from build123d import *

# Parameters (mm, degrees)
SKETCH1_R           = 1.6
BOSS_EXTRUDE1_DEPTH = 11
CUT_EXTRUDE1_DEPTH  = 6


with BuildPart() as part:
    # Sketch1 → Boss-Extrude1 (new body)
    with BuildSketch(Plane(origin=(0, 0, 0), x_dir=(1, 0, 0), z_dir=(0, 1, 0))):
        with BuildLine():
            Line((-4.5, -3.6), (4.5, -3.6))
            ThreePointArc((4.5, -3.6), (5.560660172, -3.160660172), (6, -2.1))
            Line((6, -2.1), (6, 2.1))
            ThreePointArc((6, 2.1), (5.560660172, 3.160660172), (4.5, 3.6))
            Line((4.5, 3.6), (-4.5, 3.6))
            ThreePointArc((-4.5, 3.6), (-5.560660172, 3.160660172), (-6, 2.1))
            Line((-6, 2.1), (-6, -2.1))
            ThreePointArc((-6, -2.1), (-5.560660172, -3.160660172), (-4.5, -3.6))
        make_face()
        with Locations((3, 0)):
            Circle(SKETCH1_R, mode=Mode.SUBTRACT)
    extrude(amount=-BOSS_EXTRUDE1_DEPTH)

    # Sketch2 → Cut-Extrude1 (cut)
    with BuildSketch(Plane.ZY.offset(6)):
        Polygon((-0.333384704, -11), (1.1, -11), (1.1, 0), (-0.8, 0), (-0.1, -0.45), (-0.1, -0.85), (-0.8, -1.3), (-0.8, -1.65), (-0.8, -1.999993395), (-0.1, -2.449993395), (-0.1, -2.849993395), (-0.8, -3.299993395), (-0.8, -3.64998679), (-0.8, -3.99998679), (-0.1, -4.44998679), (-0.1, -4.84998679), (-0.8, -5.29998679), (-0.8, -5.649980186), (-0.8, -5.999980186), (-0.1, -6.449980186), (-0.1, -6.849980186), (-0.8, -7.299980186), (-0.8, -7.649973581), (-0.8, -7.999973581), (-0.1, -8.449973581), (-0.1, -8.849973581), (-0.8, -9.299973581), (-0.8, -9.649966976), (-0.8, -9.999966976), (-0.1, -10.449966976), (-0.1, -10.849966976), align=None)
    extrude(amount=-CUT_EXTRUDE1_DEPTH, mode=Mode.SUBTRACT)


solid = part.part
Can you work these out from the model? Positions are in its coordinate system, mm. A direction names the side the tool comes from. Coordinates: 2 decimals unless noted, no trailing zeros. Write each loop counter-clockwise with the first axis right and the second up, starting at its lowest first coordinate (ties: lowest second). Pieces come first, ordered by that corner, then holes. Notation, with made-up numbers: (54, 52.5) - (91, 52.5) arc R18 ccw to (91, 81.5) - close; hole circle Ø9 at (15, 52.5). An arc over 180 degrees is marked (long way). Return JSON: item names as keys, results as strings. Group by question number.
Item 1: If we section it at B-B (y = -3.5): Write out the boundary of the cut face in (x, z), then the cut area to 3 significant figures.
Item 2: I'm going to push a flat-ended pin straight in: pin 1 Ø1.9 at (x, z) = (3, 0) entering from +Y. Where does the tip first touch, or does it pass through?
Item 3: If we section it at C-C (z = 1.25): Write out the boundary of the cut face in (x, y).
Item 4: We'd pull the mould along Z, two halves only. Please class faces 3 (the face through (5.55, -5.42, 3.17)), 4 (the face through (5.57, -5.42, -3.15)), 5 (the face through (0, -5, 0)): pulls with the +Z half, pulls with the -Z half, needs draft (parallel to the pull), parting line crosses it, or undercut.
Item 5: Please list where these lines run through material, in increasing order: probe 1 along X at (y, z) = (-5.5, 0); probe 2 along Z at (x, y) = (-4, -3.5); probe 3 along Z at (x, y) = (3, -5.5).
Item 6: If we section it at D-D (x = 3): Write out the boundary of the cut face in (y, z).
Item 7: Which directions (+Z, -Z, +X, -X, +Y, -Y) give clear straight access to the entire face, cutting with the end or side of a thin tool? Please do faces 1 (the face through (-3, -6, 1.1)), 2 (the face through (0, -5, 3.6)).
Return value:
{
 "1": {"outline": "(-6, -2.1) arc R1.5 ccw to (-4.5, -3.6) - (4.5, -3.6) arc R1.5 ccw to (6, -2.1) - (6, 2.1) arc R1.5 ccw to (4.5, 3.6) - (-4.5, 3.6) arc R1.5 ccw to (-6, 2.1) - (-6, 1.1) - (0, 1.1) - (0, -0.8) - (-6, -0.8) - close; hole circle Ø3.2 at (3, 0)", "area": "65.0 mm^2"},
 "2": {"pin 1": "passes through"},
 "3": {"outline": "(-6, -11) - (2, -11) - (2, 0) - (-6, 0) - close; (4, -11) - (6, -11) - (6, 0) - (4, 0) - close"},
 "4": {"face 3": "pulls with the +Z half", "face 4": "pulls with the -Z half", "face 5": "undercut"},
 "5": {"probe 1": "x = 0 to 1.4, 4.6 to 6", "probe 2": "z = -3.6 to -0.8, 1.1 to 3.6", "probe 3": "z = -3.6 to -1.6, 1.6 to 3.6"},
 "6": {"outline": "(-11, -3.6) - (0, -3.6) - (0, -1.6) - (-11, -1.6) - close; (-11, 1.6) - (0, 1.6) - (0, 3.6) - (-11, 3.6) - close"},
 "7": {"face 1": "-X, +Y, -Y", "face 2": "+Z, +X, -X, +Y, -Y"}
}
